Read the model definition and answer for the solid it produces. Units are mm, in the model's axes. A direction names the side the tool comes from. Give positions to 0.01 mm unless a question says otherwise; leave off trailing zeros. Write each loop counter-clockwise with the first axis right and the second up, starting at its lowest first coordinate (ties: lowest second). Pieces come first, ordered by that corner, then holes. Notation, with made-up numbers: (-39, 14) - (3, 14) arc R25 cw to (3, 27) - close; hole circle Ø6 at (19, 88.25). An arc over 180 degrees is marked (long way). Answer as a JSON object with one key per item and string values. Group by question number.
Autodesk Inventor part; units mm, degrees
ref_plane "YZ Plane" through (0, 0, 0) normal (1, 0, 0) x (0, 1, 0)
ref_plane "XZ Plane" through (0, 0, 0) normal (0, 1, 0) x (-1, 0, 0)
ref_plane "XY Plane" through (0, 0, 0) normal (0, 0, 1) x (1, 0, 0)
sketch "Sketch1" plane through (0, 0, 0) normal (0, 0, 1) x (1, 0, 0)
  line L0 (0, 26.67) -> (26.67, 26.67)
  line L1 (26.67, 26.67) -> (26.67, 0)
  line L2 (26.67, 0) -> (0, 0)
  line L3 (0, 0) -> (0, 26.67)
  line L4 (47.835, -21.165) -> (47.835, 47.835)
  line L5 (47.835, 47.835) -> (-21.165, 47.835)
  line L6 (-21.165, 47.835) -> (-21.165, -21.165)
  line L7 (-21.165, -21.165) -> (47.835, -21.165)
  dimension "d0" = 26.67
  dimension "d16" = 69
extrude "Extrusion1" add sketch "Sketch1" along normal blind 2
sketch "Sketch2" plane through (0, 0, 2) normal (0, 0, 1) x (1, 0, 0)
  circle A0 centre (4.835, 38.835) radius 8.0375
  circle A1 centre (-12.165, 38.835) radius 8.0375
  circle A2 centre (21.835, 38.835) radius 8.0375
  circle A3 centre (38.835, 38.835) radius 8.0375
  line L0 (47.835, 47.835) -> (-21.165, 47.835)
  line L1 (-21.165, 47.835) -> (-21.165, -21.165)
  circle A4 centre (-12.165, 21.835) radius 8.0375
  circle A5 centre (-12.165, 4.835) radius 8.0375
  circle A6 centre (38.835, 21.835) radius 8.0375
  circle A7 centre (38.835, 4.835) radius 8.0375
  circle A8 centre (4.835, -12.165) radius 8.0375
  circle A9 centre (-12.165, -12.165) radius 8.0375
  circle A10 centre (21.835, -12.165) radius 8.0375
  circle A11 centre (38.835, -12.165) radius 8.0375
  line L2 (47.835, -21.165) -> (47.835, 47.835)
  line L3 (-21.165, -21.165) -> (47.835, -21.165)
  line L4 (0, 0) -> (0, 26.67)
  line L5 (0, 26.67) -> (26.67, 26.67)
  line L6 (26.67, 26.67) -> (26.67, 0)
  line L7 (26.67, 0) -> (0, 0)
  point P0 (48.835, 48.835)
  point P1 (-20.165, 48.835)
  dimension "d4" = 16.075
  dimension "d5" = 16.075
  dimension "d6" = 16.075
  dimension "d7" = 16.075
  dimension "d8" = 9
  dimension "d9" = 9
  dimension "d10" = 9
  dimension "d11" = 9
  dimension "d12" = 9
  dimension "d13" = 17
  dimension "d14" = 17
  dimension "d15" = 17
  dimension "d17" = 16.075
  dimension "d18" = 16.075
  dimension "d19" = 16.075
  dimension "d20" = 16.075
  dimension "d21" = 16.075
  dimension "d22" = 16.075
  dimension "d23" = 16.075
  dimension "d24" = 16.075
  dimension "d25" = 17
  dimension "d26" = 17
  dimension "d27" = 17
  dimension "d28" = 17
  dimension "d29" = 17
  dimension "d30" = 17
  dimension "d31" = 17
  dimension "d32" = 17
  dimension "d33" = 17
  dimension "d34" = 9
  dimension "d35" = 9
  dimension "d36" = 9
  dimension "d37" = 9
  dimension "d38" = 9
  dimension "d39" = 9
  dimension "d40" = 9
extrude "Extrusion2" add sketch "Sketch2" along normal blind 177.8
sketch "Sketch3" plane through (0, 0, 179.8) normal (0, 0, 1) x (1, 0, 0)
  circle A0 centre (-3, 29.67) radius 2.25
  circle A1 centre (29.67, 29.67) radius 2.25
  circle A2 centre (29.67, -3) radius 2.25
  circle A3 centre (-3, -3) radius 2.25
  line L0 (0, 0) -> (0, 26.67)
  line L1 (0, 26.67) -> (26.67, 26.67)
  line L2 (26.67, 26.67) -> (26.67, 0)
  line L3 (26.67, 0) -> (0, 0)
  dimension "d43" = 4.5
  dimension "d44" = 3
  dimension "d45" = 3
  dimension "d46" = 3
  dimension "d47" = 3
  dimension "d48" = 3
  dimension "d49" = 3
  dimension "d50" = 3
  dimension "d51" = 3
extrude "Extrusion3" cut sketch "Sketch3" against normal blind 15 contours A0 | A1 | A2 | A3
fillet "Fillet1" radius 5 4 edges at (-21.165, -21.165, 89.9) (-21.165, 47.835, 89.9) (47.835, 47.835, 89.9) (47.835, -21.165, 89.9)
properties part number "WeightHolder"
1) Find section A-A, the plane x = 7. Write down the section's boundary in (y, z) (3 decimals), and give its area (3 significant figures).
2) Flat-ended cylindrical pins translate along their axes: pin 1 Ø1.3 at (x, y) = (29.5, -3.5) entering from +Z; pin 2 Ø5 at (x, y) = (35, 42) entering from +Z. Find the tip coordinate at first contact, or state that the pin passes through.
3) Find section C-C, the plane z = 166.5. Give the number of separate pieces and of enclosed holes in the cut face, and give its area (3 significant figures).
4) Which of the six approach directions +Z, -Z, +X, -X, +Y, -Y give full straight-line access (tool end or side, diameter ignored) to faces 5 (the cylindrical face through (-3.488, 27.474, 172.405)), 6 (the flat face through (-21.165, 14, 89))?
5) For a pull along Y with two mould halves and no side action, classify faces 1 (the flat face through (39, -12, 2)), 2 (the flat face through (14, 47.835, 89)), 3 (the cylindrical face through (46.33, -19.74, 91.16)), 4 (the cylindrical face through (31.816, -2.324, 172.405)) as released by +Y, released by -Y, zero draft, split by the parting line, or undercut.
6) Find the intervals of material crossed by line 1 (X direction, y = -6.5, z = 117.5) (3 decimals); line 2 (Y direction, x = -16, z = 54) (3 decimals); line 3 (Y direction, x = 16.5, z = 121) (3 decimals), in increasing order. Write a range as [from, to].
Values follow:
{
 "1": {"outline": "(-21.165, 0) - (0, 0) - (0, 179.8) - (-4.425, 179.8) - (-4.425, 2) - (-19.905, 2) - (-19.905, 179.8) - (-21.165, 179.8) - close; (26.67, 0) - (47.835, 0) - (47.835, 179.8) - (46.575, 179.8) - (46.575, 2) - (31.095, 2) - (31.095, 179.8) - (26.67, 179.8) - close", "area": "2,110 mm2"},
 "2": {"pin 1": "stops at z = 164.8", "pin 2": "stops at z = 2"},
 "3": {"separate pieces": "1", "enclosed holes": "17", "area": "1,530 mm2"},
 "4": {"face 5": "+Z", "face 6": "+Z, -Z, -X, +Y, -Y"},
 "5": {"face 1": "undercut", "face 2": "released by +Y", "face 3": "released by -Y", "face 4": "undercut"},
 "6": {"line 1": "x = [-21.165, -17.867], [-6.463, -0.867], [10.537, 16.133], [27.537, 33.133], [44.537, 47.835]", "line 2": "y = [-21.165, -19.229], [-5.101, -2.229], [11.899, 14.771], [28.899, 31.771], [45.899, 47.835]", "line 3": "y = [-21.165, -18.177], [-6.153, 0], [26.67, 32.823], [44.847, 47.835]"}
}
